Can you work these out from the model? Positions are in its coordinate system, mm. A direction names the side the tool comes from. Coordinates: 2 decimals unless noted, no trailing zeros. Order: outer loops, then holes, each group sorted by start corner. A loop starts at its lowest first (then second) coordinate and runs counter-clockwise, first axis right, second up.
```python
from build123d import *

# Parameters (mm, degrees)
SKETCH1_R           = 75
BOSS_EXTRUDE1_DEPTH = 200
BOSS_EXTRUDE1_TAPER = 5
SKETCH2_R           = 75
BOSS_EXTRUDE2_DEPTH = 20
SHELL2_T            = -1
CUT_EXTRUDE1_REACH  = 228.385
SKETCH3_R           = 3.75
CIRPATTERN1_COUNT   = 5


with BuildPart() as part:
    # Sketch1 → Boss-Extrude1 (new body)
    with BuildSketch(Plane(origin=(0, 0, 0), x_dir=(1, 0, 0), z_dir=(0, 1, 0))):
        Circle(SKETCH1_R)
    extrude(amount=BOSS_EXTRUDE1_DEPTH, taper=BOSS_EXTRUDE1_TAPER)

    # Sketch2 → Boss-Extrude2 (add)
    with BuildSketch(Plane(origin=(0, 0, 0), x_dir=(1, 0, 0), z_dir=(0, 1, 0))):
        with Locations(Location((0, 0, 0), (0, 0, 270))):
            Circle(SKETCH2_R)
    extrude(amount=BOSS_EXTRUDE2_DEPTH)

    # Shell2
    shell2_openings = [part.faces().sort_by_distance(p)[0] for p in [
        (0, 0, 0),
    ]]
    offset(amount=SHELL2_T, openings=shell2_openings, kind=Kind.INTERSECTION)

    # Sketch3 → Cut-Extrude1 (cut, up to next)
    with BuildSketch(Plane(origin=(0, 200, 0), x_dir=(1, 0, 0), z_dir=(0, 1, 0)), mode=Mode.PRIVATE) as cut_extrude1_sk1:
        with Locations(Location((0, 35, 0), (0, 0, 270))):
            Circle(SKETCH3_R)
    cut_extrude1_tool1 = extrude(cut_extrude1_sk1.sketch, amount=-CUT_EXTRUDE1_REACH, mode=Mode.PRIVATE) & part.part
    cut_extrude1 = cut_extrude1_tool1.solids().sort_by_distance((0, 200, -35))[0]
    add(cut_extrude1, mode=Mode.SUBTRACT)

    # CirPattern1: Cut-Extrude1 ×5 about axis
    cirpattern1_axis = Axis((0, 0, 0), (0, 1, 0))
    for i in range(1, CIRPATTERN1_COUNT):
        add(cut_extrude1.rotate(cirpattern1_axis, i * 360 / CIRPATTERN1_COUNT), mode=Mode.SUBTRACT)


solid = part.part
```
1. Please list where these lines run through material, in increasing order: probe 1 along X at (y, z) = (10.25, 0); probe 2 along Y at (x, z) = (-53.5, -2); probe 3 along Z at (x, y) = (-46, 91.5).
Completed:
probe 1: x = -75 to -74, 74 to 75
probe 2: y = 199 to 200
probe 3: z = -48.71 to -47.32, 47.32 to 48.71
2. Imagine slicing it at A-A on y = 100. Please give me the cut outline in (x, z).
Completed:
outline: circle Ø132.5 at (0, 0); hole circle Ø130.49 at (0, 0)
3. Imagine slicing it at B-B on y = 122. Please give me the cut outline in (x, z), then the cut area to 3 significant figures.
Completed:
outline: circle Ø128.65 at (0, 0); hole circle Ø126.65 at (0, 0)
area: 403 mm2
4. On a 3-axis mill with a long thin cutter (end or side, diameter ignored), from which of +Z, -Z, +X, -X, +Y, -Y can I reach the whole of each face in a straight line? I mean faces 5 (the flat face through (-72, 20, 16)), 6 (the flat face through (55, 0, 50)), 7 (the flat face through (-1, 199, -1)). Say none if no direction works.
Completed:
face 5: +Y
face 6: +Z, -Z, +X, -X, -Y
face 7: -Y
5. I'm going to push flat-ended pins straight in: pin 1 (1 mm diameter, centred on y = 30.5, z = -54.5, fed in from -X); pin 2 (8 mm diameter, centred on x = 19.5, z = -23.5, fed in from -Y); pin 3 (5 mm diameter, centred on x = -17.5, y = 149.5, fed in from -Z). Where does each tip first touch, or does it pass through?
Completed:
pin 1: stops at x = -48.13
pin 2: stops at y = 199
pin 3: stops at z = -60.12
6. Thinking about a two-plate mould opening in X: for faces 1 (the cylindrical face through (-45.636, 9.86, -59.517)), 2 (the cylindrical face through (-30.393, 199.507, -13.2)), 3 (the flat face through (-1, 200, -1)), 4 (the cylindrical face through (-28.34, 9.37, 68.36)), which applies, pulls with the +X half, pulls with the -X half, needs draft (parallel to the pull), parting line crosses it, or undercut?
Completed:
face 1: parting line crosses it
face 2: undercut
face 3: needs draft
face 4: undercut
